Source: CAD feature listing. Evaluate the final solid. Frame: model axes, mm. A direction names the side the tool comes from. Round coordinates to 2 decimals unless told otherwise and drop trailing zeros. Loops run counter-clockwise (first coordinate to the right, second up) from the corner with the lowest first, then second, coordinate; pieces in that order, holes last.
Item 1: Section query B-B on x = 0. Return loops of the section in (y, z).
Item 2: Section query A-A on y = 14.75. Return loops of the section in (x, z), then the cut area to 3 significant figures.
Item 3: Section query C-C on x = -12.5. Return loops of the section in (y, z), then the cut area to 3 significant figures.
Item 4: First-contact query: P1, Ø2, axis at x = -15, y = 21.5, coming from the -Z side; P2, Ø3, axis at x = -1.5, y = 16, coming from the +Z side; P3, Ø2, axis at x = -15.5, y = 22.5, coming from the +Z side. Flat tips, straight axial feed; report the tip coordinate or a pass-through.
Item 5: Pull-direction query (Z, two-part tool) for faces 1 (the flat face through (16.8, 26, -21.4)), 2 (the flat face through (8.187, 11.339, 21.099)); classes: released by +Z, released by -Z, zero draft, split by the parting line, or undercut.
Item 6: Ray query, L1, parallel to X at y = 24.65, z = 0; L2, parallel to Z at x = -19, y = 24.75; L3, parallel to Y at x = -8.5, z = 21.5. Return the intervals inside material, ascending.
Item 7: Access query for faces 3 (the flat face through (-8.163, 11.339, 21.124)), 4 (the cylindrical face through (0.99, 24.48, -24.98)), 5 (the flat face through (0, 0, -7)). Directions: +Z, -Z, +X, -X, +Y, -Y. A direction counts if a zero-diameter tool reaches every point of the face in a straight line with its end or side. Return the directions, or none.
Item 8: Section query D-D on z = 17. Return loops of the section in (x, y).
```python
from build123d import *
from build123d.topology import SkipClean

# Parameters (mm, degrees)
SKETCH1_R           = 28.5
BOSS_EXTRUDE1_DEPTH = 3
BOSS_EXTRUDE4_DEPTH = 20
BOSS_EXTRUDE7_DEPTH = 3
CUT_EXTRUDE1_START  = -2
CUT_EXTRUDE1_DEPTH  = 2
CUT_EXTRUDE5_START  = -4
CUT_EXTRUDE5_DEPTH  = 4


# Read off the part's stored shape, not the designer's step: Boss-Extrude7
with BuildPart() as part:
    # Sketch1 → Boss-Extrude1 (new body)
    with BuildSketch(Plane(origin=(0, 0, 0), x_dir=(1, 0, 0), z_dir=(0, 1, 0))):
        with Locations(Location((0, 0, 0), (0, 0, 270))):
            Circle(SKETCH1_R)
    extrude(amount=BOSS_EXTRUDE1_DEPTH)

    # Sketch2 → Boss-Extrude4 (add)
    with BuildSketch(Plane(origin=(0, 3, 0), x_dir=(1, 0, 0), z_dir=(0, 1, 0))):
        with BuildLine():
            Line((-9, -20.223805295), (-9, -18.723805295))
            ThreePointArc((-9, -18.723805295), (-11.855740218, -15.445899804), (-13.568253388, -11.45))
            ThreePointArc((-13.568253388, -11.45), (-14, -8), (-13.568253388, -4.55))
            ThreePointArc((-13.568253388, -4.55), (0, 6), (13.568253388, -4.55))
            ThreePointArc((13.568253388, -4.55), (14, -8), (13.568253388, -11.45))
            ThreePointArc((13.568253388, -11.45), (11.855740218, -15.445899804), (9, -18.723805295))
            Line((9, -18.723805295), (9, -20.223805295))
            Line((9, -20.223805295), (7.35, -22))
            Line((7.35, -22), (7.617272727, -27.463196394))
            ThreePointArc((7.617272727, -27.463196394), (22.686364547, -17.250474302), (28.5, 0))
            ThreePointArc((28.5, 0), (-17.250474302, 22.686364547), (-7.617272727, -27.463196394))
            Line((-7.617272727, -27.463196394), (-7.35, -22))
            Line((-7.35, -22), (-9, -20.223805295))
        make_face()
    extrude(amount=BOSS_EXTRUDE4_DEPTH)

    # Boss-Extrude7 outline → Boss-Extrude7 (add)
    with BuildSketch(Plane(origin=(0, 23, 0), x_dir=(1, 0, 0), z_dir=(0, 1, 0))):
        with BuildLine():
            ThreePointArc((7.617272727, -27.463196394), (0, 28.5), (-7.617272727, -27.463196394))
            Line((-7.617272727, -27.463196394), (-7.542031899, -25.92523394))
            ThreePointArc((-7.542031899, -25.92523394), (0, 27), (7.542031899, -25.92523394))
            Line((7.542031899, -25.92523394), (7.617272727, -27.463196394))
        make_face()
        with BuildLine():
            ThreePointArc((7.441330866, -23.866851383), (0, 25), (-7.441330866, -23.866851383))
            Line((-7.441330866, -23.866851383), (-7.365455329, -22.315915124))
            ThreePointArc((-7.365455329, -22.315915124), (0, 23.5), (7.365455329, -22.315915124))
            Line((7.365455329, -22.315915124), (7.441330866, -23.866851383))
        make_face()
    extrude(amount=BOSS_EXTRUDE7_DEPTH)

    # Sketch6 → Cut-Extrude1 (cut)
    with SkipClean():  # the faces are left unmerged after this step: merging them gives an invalid solid
        with BuildSketch(Plane(origin=(0, 23, 0), x_dir=(1, 0, 0), z_dir=(0, 1, 0)).offset(CUT_EXTRUDE1_START)):
            with BuildLine():
                Line((13.568253388, -11.45), (17.5, -11.45))
                ThreePointArc((17.5, -11.45), (20.95, -8), (17.5, -4.55))
                Line((17.5, -4.55), (13.568253388, -4.55))
                ThreePointArc((13.568253388, -4.55), (0, 6), (-13.568253388, -4.55))
                Line((-13.568253388, -4.55), (-17.5, -4.55))
                ThreePointArc((-17.5, -4.55), (-20.95, -8), (-17.5, -11.45))
                Line((-17.5, -11.45), (-13.568253388, -11.45))
                ThreePointArc((-13.568253388, -11.45), (-11.855740218, -15.445899804), (-9, -18.723805295))
                Line((-9, -18.723805295), (-9, -20.223805295))
                Line((-9, -20.223805295), (-7.35, -22))
                Line((-7.35, -22), (-7.35, -25))
                Line((-7.35, -25), (7.35, -25))
                Line((7.35, -25), (7.35, -22))
                Line((7.35, -22), (9, -20.223805295))
                Line((9, -20.223805295), (9, -18.723805295))
                ThreePointArc((9, -18.723805295), (11.855740218, -15.445899804), (13.568253388, -11.45))
            make_face()
        extrude(amount=CUT_EXTRUDE1_DEPTH, mode=Mode.SUBTRACT)

    # Sketch7 → Cut-Extrude5 (cut)
    with BuildSketch(Plane(origin=(0, 3, 0), x_dir=(1, 0, 0), z_dir=(0, 1, 0)).offset(CUT_EXTRUDE5_START)):
        with BuildLine():
            Line((-9, -20.223805295), (-7.35, -22))
            Line((-7.35, -22), (-7.617272727, -27.463196394))
            ThreePointArc((-7.617272727, -27.463196394), (0, -28.5), (7.617272727, -27.463196394))
            Line((7.617272727, -27.463196394), (7.35, -22))
            Line((7.35, -22), (9, -20.223805295))
            Line((9, -20.223805295), (9, -18.723805295))
            ThreePointArc((9, -18.723805295), (0, 6), (-9, -18.723805295))
            Line((-9, -18.723805295), (-9, -20.223805295))
        make_face()
    extrude(amount=CUT_EXTRUDE5_DEPTH, mode=Mode.SUBTRACT)


solid = part.part
```
Data:
1. outline: (0, -28.5) - (26, -28.5) - (26, -27) - (23, -27) - (23, -25) - (26, -25) - (26, -23.5) - (23, -23.5) - (23, -6) - (0, -6) - close
2. outline: (-9, 18.72) - (-9, 20.22) - (-7.35, 22) - (-7.62, 27.46) arc R28.5 ccw (long way) to (7.62, 27.46) - (7.35, 22) - (9, 20.22) - (9, 18.72) arc R14 cw (long way) to start
2. area: 1,830 mm2
3. outline: (0, -25.61) - (26, -25.61) - (26, -23.93) - (23, -23.93) - (23, -21.65) - (26, -21.65) - (26, -19.9) - (23, -19.9) - (23, 1.7) - (0, 1.7) - close; (0, 14.3) - (23, 14.3) - (23, 19.9) - (26, 19.9) - (26, 21.65) - (23, 21.65) - (23, 23.93) - (26, 23.93) - (26, 25.61) - (0, 25.61) - close
3. area: 909 mm2
4. P1: stops at z = -24.82
4. P2: stops at z = -5.67
4. P3: stops at z = 24.54
5. face 1: zero draft
5. face 2: undercut
6. L1: x = -28.5 to -27, -25 to -23.5, 23.5 to 25, 27 to 28.5
6. L2: z = -21.24 to -19.18, -16.25 to -13.83, 13.83 to 16.25, 19.18 to 21.24
6. L3: y = 0 to 23
7. face 3: +Y, -Y
7. face 4: +Y
7. face 5: +Z, -Z, +X, -X, -Y
8. outline: (-22.87, 0) - (-10.72, 0) - (-10.72, 23) - (-16.22, 23) - (-16.22, 26) - (-18.33, 26) - (-18.33, 23) - (-20.98, 23) - (-20.98, 26) - (-22.87, 26) - close; (10.72, 0) - (22.87, 0) - (22.87, 26) - (20.98, 26) - (20.98, 23) - (18.33, 23) - (18.33, 26) - (16.22, 26) - (16.22, 23) - (10.72, 23) - close
